Read the model definition and answer for the solid it produces. Units are mm, in the model's axes. Give positions to 0.01 mm unless a question says otherwise; leave off trailing zeros. Loops run counter-clockwise (first coordinate to the right, second up) from the corner with the lowest first, then second, coordinate; pieces in that order, holes last. Notation, with made-up numbers: (-27, 12.25) - (-3, 12.25) arc R13 cw to (-3, 29.25) - close; hole circle Ø2 at (2.25, 20.5). An arc over 180 degrees is marked (long way). Put each result on its own line as item: value. Start each with the question number.
1. A cutting plane is placed at C-C, the plane z = 50. Determine the outline of the cut face in (x, y).
2. A cutting plane is placed at B-B, the plane y = 199.5. Determine the outline of the cut face in (x, z), plus the area to 3 significant figures.
3. Given pin 1 Ø1.5 at (y, z) = (189, 721.5) entering from +X; pin 2 Ø24 at (y, z) = (93.5, 50) entering from +X; pin 3 Ø7.5 at (x, y) = (288.5, 3) entering from -Z, each flat-ended and moving along its own axis, determine where each tip first touches the part or whether it passes through.
4. Consider L1, parallel to X at y = -218, z = 488.5; L2, parallel to Z at x = 292.5, y = 129.5; L3, parallel to X at y = -263, z = 60. Determine where each line is inside the solid, lowest interval first. Write a range as from..to.
5. A cutting plane is placed at A-A, the plane y = 69. Determine the outline of the cut face in (x, z).
```python
from build123d import *

# Parameters (mm, degrees)
F0_W          = 600
F0_H          = 600
F1_DEPTH      = 800
F2_W          = 600
F2_H          = 80
F3_DEPTH      = 25
F4_W          = 630
F4_H          = 600
F5_DEPTH      = 25
F7_DEPTH      = 50
F8_W          = 40
F8_H          = 180
F9_DEPTH      = 25
F10_T1_DEPTH  = 190
F10_T4_ANGLE  = 180
F10_T8_DEPTH  = 52.5
F10_S9_R      = 5
F10_T10_DEPTH = 28
F10_T14_DEPTH = 205
F10_S15_R     = 5
F10_T16_DEPTH = 104
F10_S17_R     = 5
F10_T18_DEPTH = 104
F10_T22_DEPTH = 52.5
F10_S23_R     = 5
F10_T24_DEPTH = 28
F10_T28_DEPTH = 52.5
F10_S29_R     = 5
F10_T30_DEPTH = 28
F10_T34_DEPTH = 205
F10_S35_R     = 5
F10_T36_DEPTH = 104
F10_S37_R     = 5
F10_T38_DEPTH = 104
F10_T42_DEPTH = 52.5
F10_S43_R     = 5
F10_T44_DEPTH = 28
F10_T46_ANGLE = 180


# Not quite as in the source:
# - a fillet or chamfer that OpenCascade refuses, or shapes differently, is made with other operations: its cross-section is extruded or revolved along the edge and cut away or added


with BuildPart() as f1:
    # F0 (on Top) → F1 (new body)
    with BuildSketch(Plane.XY):
        Rectangle(F0_W, F0_H)
    extrude(amount=F1_DEPTH)

    # F2 (on face) → F3 (cut)
    with BuildSketch(Plane.YZ.offset(300)):
        with Locations((0, 40)):
            Rectangle(F2_W, F2_H)
    extrude(amount=-F3_DEPTH, mode=Mode.SUBTRACT)

    # F4 (on face) → F5 (join)
    with BuildSketch(Plane.XY.offset(800)):
        with Locations((15, 0)):
            Rectangle(F4_W, F4_H)
    extrude(amount=F5_DEPTH)

    # F6 (on face) → F7 (join)
    with BuildSketch(Plane.YZ.offset(300)):
        with BuildLine():
            ThreePointArc((100, 749.2423057556), (98.5355339059, 752.7778396615), (95, 754.2423057556))
            Line((95, 754.2423057556), (-95, 754.2423057556))
            ThreePointArc((-95, 754.2423057556), (-98.5355339059, 752.7778396615), (-100, 749.2423057556))
            ThreePointArc((-100, 749.2423057556), (-98.5355339059, 745.7067718497), (-95, 744.2423057556))
            Line((-95, 744.2423057556), (95, 744.2423057556))
            ThreePointArc((95, 744.2423057556), (98.5355339059, 745.7067718497), (100, 749.2423057556))
        make_face()
    extrude(amount=F7_DEPTH)

    # F8 (on face) → F9 (cut)
    with BuildSketch(Plane(origin=(0, 0, 744.2423057556), x_dir=(1, 0, 0), z_dir=(0, 0, -1))):
        with Locations((320, 0)):
            Rectangle(F8_W, F8_H)
    extrude(amount=-F9_DEPTH, mode=Mode.SUBTRACT)

    # F10: fillet of radius 5 on 10 edges, made by hand

    # F10_s2 → F10_t1 (cut)
    with BuildSketch(Plane.XZ.offset(-95)):
        with BuildLine():
            ThreePointArc((345, 754.2423057556), (348.5355339059, 752.7778396615), (350, 749.2423057556))
            Line((350, 749.2423057556), (350, 754.2423057556))
            Line((350, 754.2423057556), (345, 754.2423057556))
        make_face()
        with BuildLine():
            ThreePointArc((345, 744.2423057556), (348.5355339059, 745.7067718497), (350, 749.2423057556))
            Line((350, 749.2423057556), (350, 744.2423057556))
            Line((350, 744.2423057556), (345, 744.2423057556))
        make_face()
    extrude(amount=F10_T1_DEPTH, mode=Mode.SUBTRACT)

    # F10_s3 → F10_t4 (revolve, cut)
    with BuildSketch(Plane.XZ.offset(-95)):
        with BuildLine():
            ThreePointArc((345, 754.2423057556), (348.5355339059, 752.7778396615), (350, 749.2423057556))
            Line((350, 749.2423057556), (350, 754.2423057556))
            Line((350, 754.2423057556), (345, 754.2423057556))
        make_face()
    revolve(axis=Axis((350, 95, 749.2423057556), (-1, 0, 0)), revolution_arc=F10_T4_ANGLE, mode=Mode.SUBTRACT)


with BuildPart() as f10_tool6:
    # F10_s7 → F10_t8 (new body)
    with BuildSketch(Plane.YZ.offset(300)):
        with BuildLine():
            ThreePointArc((95, 744.2423057556), (91.4644660941, 745.7067718497), (90, 749.2423057556))
            Line((90, 749.2423057556), (90, 744.2423057556))
            Line((90, 744.2423057556), (95, 744.2423057556))
        make_face()
    extrude(amount=F10_T8_DEPTH)

    # F10_s9 → F10_t10 (cut, symmetric)
    with BuildSketch(Plane.XZ.offset(-92.5)):
        with Locations((345, 749.2423057556)):
            Circle(F10_S9_R)
    extrude(amount=F10_T10_DEPTH, both=True, mode=Mode.SUBTRACT)


with BuildPart() as f1_1:
    add(f1.part)

    # F10_t5: cut F10_tool6
    add(f10_tool6.part, mode=Mode.SUBTRACT)


with BuildPart() as f10_tool12:
    # F10_s13 → F10_t14 (new body)
    with BuildSketch(Plane.XZ.offset(-102.5)):
        with BuildLine():
            ThreePointArc((345, 744.2423057556), (341.4644660941, 745.7067718497), (340, 749.2423057556))
            Line((340, 749.2423057556), (340, 744.2423057556))
            Line((340, 744.2423057556), (345, 744.2423057556))
        make_face()
    extrude(amount=F10_T14_DEPTH)

    # F10_s15 → F10_t16 (cut, symmetric)
    with BuildSketch(Plane.YZ.offset(342.5)):
        with Locations((-95, 749.2423057556)):
            Circle(F10_S15_R)
    extrude(amount=F10_T16_DEPTH, both=True, mode=Mode.SUBTRACT)

    # F10_s17 → F10_t18 (cut, symmetric)
    with BuildSketch(Plane.YZ.offset(342.5)):
        with Locations((95, 749.2423057556)):
            Circle(F10_S17_R)
    extrude(amount=F10_T18_DEPTH, both=True, mode=Mode.SUBTRACT)


with BuildPart() as f1_2:
    add(f1_1.part)

    # F10_t11: cut F10_tool12
    add(f10_tool12.part, mode=Mode.SUBTRACT)


with BuildPart() as f10_tool20:
    # F10_s21 → F10_t22 (new body)
    with BuildSketch(Plane.YZ.offset(352.5)):
        with BuildLine():
            ThreePointArc((-95, 744.2423057556), (-91.4644660941, 745.7067718497), (-90, 749.2423057556))
            Line((-90, 749.2423057556), (-90, 744.2423057556))
            Line((-90, 744.2423057556), (-95, 744.2423057556))
        make_face()
    extrude(amount=-F10_T22_DEPTH)

    # F10_s23 → F10_t24 (cut, symmetric)
    with BuildSketch(Plane.XZ.offset(92.5)):
        with Locations((345, 749.2423057556)):
            Circle(F10_S23_R)
    extrude(amount=F10_T24_DEPTH, both=True, mode=Mode.SUBTRACT)


with BuildPart() as f1_3:
    add(f1_2.part)

    # F10_t19: cut F10_tool20
    add(f10_tool20.part, mode=Mode.SUBTRACT)


with BuildPart() as f10_tool26:
    # F10_s27 → F10_t28 (new body)
    with BuildSketch(Plane.YZ.offset(300)):
        with BuildLine():
            ThreePointArc((95, 754.2423057556), (91.4644660941, 752.7778396615), (90, 749.2423057556))
            Line((90, 749.2423057556), (90, 754.2423057556))
            Line((90, 754.2423057556), (95, 754.2423057556))
        make_face()
    extrude(amount=F10_T28_DEPTH)

    # F10_s29 → F10_t30 (cut, symmetric)
    with BuildSketch(Plane.XZ.offset(-92.5)):
        with Locations((345, 749.2423057556)):
            Circle(F10_S29_R)
    extrude(amount=F10_T30_DEPTH, both=True, mode=Mode.SUBTRACT)


with BuildPart() as f1_4:
    add(f1_3.part)

    # F10_t25: cut F10_tool26
    add(f10_tool26.part, mode=Mode.SUBTRACT)


with BuildPart() as f10_tool32:
    # F10_s33 → F10_t34 (new body)
    with BuildSketch(Plane.XZ.offset(-102.5)):
        with BuildLine():
            ThreePointArc((345, 754.2423057556), (341.4644660941, 752.7778396615), (340, 749.2423057556))
            Line((340, 749.2423057556), (340, 754.2423057556))
            Line((340, 754.2423057556), (345, 754.2423057556))
        make_face()
    extrude(amount=F10_T34_DEPTH)

    # F10_s35 → F10_t36 (cut, symmetric)
    with BuildSketch(Plane.YZ.offset(342.5)):
        with Locations((95, 749.2423057556)):
            Circle(F10_S35_R)
    extrude(amount=F10_T36_DEPTH, both=True, mode=Mode.SUBTRACT)

    # F10_s37 → F10_t38 (cut, symmetric)
    with BuildSketch(Plane.YZ.offset(342.5)):
        with Locations((-95, 749.2423057556)):
            Circle(F10_S37_R)
    extrude(amount=F10_T38_DEPTH, both=True, mode=Mode.SUBTRACT)


with BuildPart() as f1_5:
    add(f1_4.part)

    # F10_t31: cut F10_tool32
    add(f10_tool32.part, mode=Mode.SUBTRACT)


with BuildPart() as f10_tool40:
    # F10_s41 → F10_t42 (new body)
    with BuildSketch(Plane.YZ.offset(352.5)):
        with BuildLine():
            ThreePointArc((-95, 754.2423057556), (-91.4644660941, 752.7778396615), (-90, 749.2423057556))
            Line((-90, 749.2423057556), (-90, 754.2423057556))
            Line((-90, 754.2423057556), (-95, 754.2423057556))
        make_face()
    extrude(amount=-F10_T42_DEPTH)

    # F10_s43 → F10_t44 (cut, symmetric)
    with BuildSketch(Plane.XZ.offset(92.5)):
        with Locations((345, 749.2423057556)):
            Circle(F10_S43_R)
    extrude(amount=F10_T44_DEPTH, both=True, mode=Mode.SUBTRACT)


with BuildPart() as f1_6:
    add(f1_5.part)

    # F10_t39: cut F10_tool40
    add(f10_tool40.part, mode=Mode.SUBTRACT)

    # F10_s45 → F10_t46 (revolve, cut)
    with BuildSketch(Plane.XZ.offset(95)):
        with BuildLine():
            ThreePointArc((345, 744.2423057556), (348.5355339059, 745.7067718497), (350, 749.2423057556))
            Line((350, 749.2423057556), (350, 744.2423057556))
            Line((350, 744.2423057556), (345, 744.2423057556))
        make_face()
    revolve(axis=Axis((350, -95, 749.2423057556), (-1, 0, 0)), revolution_arc=F10_T46_ANGLE, mode=Mode.SUBTRACT)


solid = f1_6.part
```
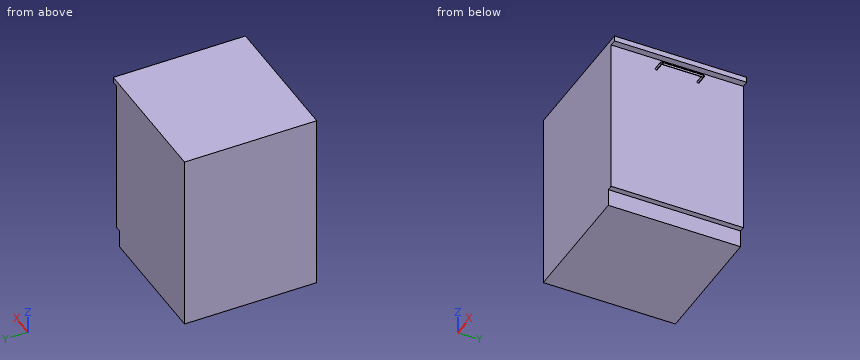
Return value:
1. outline: (-300, -300) - (275, -300) - (275, 300) - (-300, 300) - close
2. outline: (-300, 0) - (275, 0) - (275, 80) - (300, 80) - (300, 800) - (330, 800) - (330, 825) - (-300, 825) - close
2. area: 494,000 mm2
3. pin 1: stops at x = 300
3. pin 2: stops at x = 275
3. pin 3: stops at z = 80
4. L1: x = -300..300
4. L2: z = 80..825
4. L3: x = -300..275
5. outline: (-300, 0) - (275, 0) - (275, 80) - (300, 80) - (300, 800) - (330, 800) - (330, 825) - (-300, 825) - close; circle Ø10 at (345, 749.24)
